Source: CAD feature listing. Evaluate the final solid. Frame: model axes, mm. A direction names the side the tool comes from. Give positions to 0.01 mm unless a question says otherwise; leave off trailing zeros. Write each loop counter-clockwise with the first axis right and the second up, starting at its lowest first coordinate (ties: lowest second). Pieces come first, ordered by that corner, then holes. Notation, with made-up numbers: (64, -34.75) -> (85, -34.75) arc R18 ccw to (85, -24.75) -> close; hole circle Ø1 at (3.25, -28.5). An arc over 180 degrees is marked (long way). Write item = value, one per line.
from build123d import *

# Parameters (mm, degrees)
ESQUISSE1_W             = 37.1
ESQUISSE1_H             = 29.3
ESQUISSE1_R             = 1.175
BOSS_EXTRU_1_DEPTH      = 1.2
ENL_V_MAT_EXTRU_1_DEPTH = 0.01


with BuildPart() as part:
    # Esquisse1 → Boss.-Extru.1 (new body)
    with BuildSketch(Plane(origin=(0, 0, 0), x_dir=(1, 0, 0), z_dir=(0, 1, 0))):
        Rectangle(ESQUISSE1_W, ESQUISSE1_H)
        with Locations(Location((-10.375, 8.575, 0), (0, 0, 270))):
            Circle(ESQUISSE1_R, mode=Mode.SUBTRACT)
        with BuildLine():
            Line((7.15, 12.175), (7.15, 10.725))
            ThreePointArc((7.15, 10.725), (5.975, 9.55), (4.8, 10.725))
            Line((4.8, 10.725), (4.8, 12.175))
            ThreePointArc((4.8, 12.175), (5.975, 13.35), (7.15, 12.175))
        make_face(mode=Mode.SUBTRACT)
    extrude(amount=BOSS_EXTRU_1_DEPTH)

    # Esquisse2 → Enlèv. mat.-Extru.1 (cut)
    with BuildSketch(Plane(origin=(0, 1.2, 0), x_dir=(1, 0, 0), z_dir=(0, 1, 0))):
        with BuildLine():
            Line((-12.55, -4.923584906), (-9.55, -0.554374451))
            ThreePointArc((-9.55, -0.554374451), (-6.521273623, -1.1783268), (-4.851037813, -3.780789545))
            Line((-4.851037813, -3.780789545), (-7.851037813, -8.15))
            ThreePointArc((-7.851037813, -8.15), (-10.879764189, -7.52604765), (-12.55, -4.923584906))
        make_face()
        with BuildLine():
            Line((3.851037813, -5.824109363), (6.851037813, -1.454898908))
            ThreePointArc((6.851037813, -1.454898908), (9.879764189, -2.078851257), (11.55, -4.681314002))
            Line((11.55, -4.681314002), (8.55, -9.050524457))
            ThreePointArc((8.55, -9.050524457), (5.521273623, -8.426572107), (3.851037813, -5.824109363))
        make_face()
    extrude(amount=-ENL_V_MAT_EXTRU_1_DEPTH, mode=Mode.SUBTRACT)


solid = part.part
1) Contact query for flat-ended pins moving along their axis: pin 1 (6 mm diameter, centred on x = 7, z = 6, fed in from +Y); pin 2 (1.4 mm diameter, centred on x = -10.375, z = -8.575, fed in from +Y). Output: stop coordinate, or through.
Computed:
pin_1 = 1.2
pin_2 = through
2) Draft query along Z for faces 1 (the flat face through (0, 1, -14.65)), 2 (the flat face through (0, 0, 0)), 3 (the cylindrical face through (-11.4, 0.6, -8)). Return one class per face: pulls with the +Z half, pulls with the -Z half, needs draft (parallel to the pull), parting line crosses it, or undercut.
Computed:
face_1 = pulls with the -Z half
face_2 = needs draft
face_3 = undercut
3) Cut plane A-A (z = -10.25). Return the cut outline in (x, y), then the cut area to 3 significant figures.
Computed:
outline = (-18.55, 0) -> (4.9, 0) -> (4.9, 1.2) -> (-18.55, 1.2) -> close; (7.05, 0) -> (18.55, 0) -> (18.55, 1.2) -> (7.05, 1.2) -> close
area = 41.9 mm²
4) Material intervals for L1, parallel to X at y = 1, z = -8.75; L2, parallel to X at y = 0.7, z = -12.5; L3, parallel to Z at x = -9.5, y = 0.65, sorted ascending.
Computed:
L1 = -18.55 to -11.54, -9.21 to 18.55
L2 = -18.55 to 4.85, 7.1 to 18.55
L3 = -14.65 to -9.36, -7.79 to 14.65
5) Access query for faces 4 (the flat face through (0, 1, 14.65)), 5 (the cylindrical face through (5.95, 0.59, -13.35)). Directions: +Z, -Z, +X, -X, +Y, -Y. A direction counts if a zero-diameter tool reaches every point of the face in a straight line with its end or side. Return the directions, or none.
Computed:
face_4 = +Z, +X, -X, +Y, -Y
face_5 = +Y, -Y
